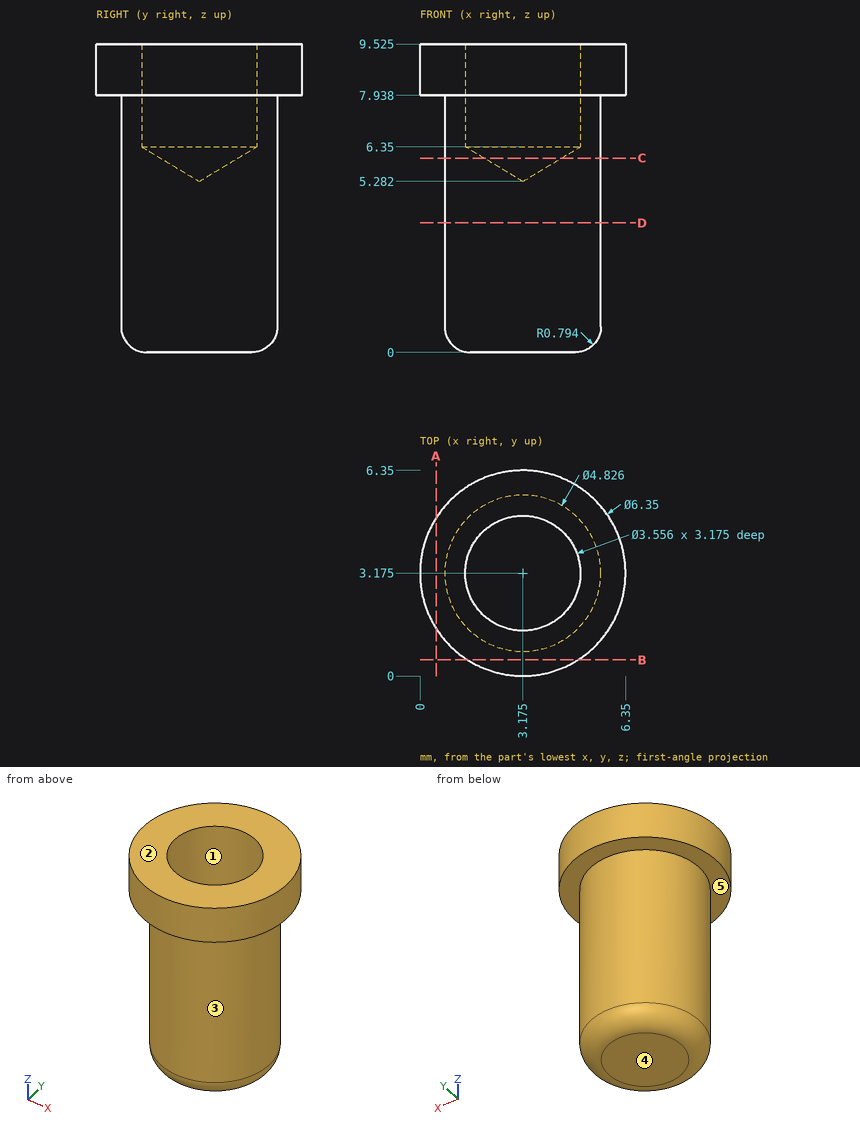
Check sheet for the drawn part. Datum: minimum x, y, z corner. Units: mm. A direction names the side the tool comes from. Round coordinates to 2 decimals unless told otherwise and drop trailing zeros. Loops run counter-clockwise (first coordinate to the right, second up) from the corner with the lowest first, then second, coordinate; pieces in that order, holes last. Notation, with made-up numbers: (-4.75, 58) - (52.25, 58) arc R16 cw to (52.25, 75) - close; hole circle Ø7 at (75.25, 35.25). An arc over 180 degrees is marked (long way). Write item = value, one per line. Start each with the question number.
1. Set-up check for the marked faces 4 and 5: record each of +Z, -Z, +X, -X, +Y, -Y from which the full face is reachable in a straight line by a thin tool's end or side.
2. Section check D-D on z = 4. Enter the section's corners in (x, y) (1 decimal).
3. Mould release check, pull along Y, two halves, no side actions. Record for the marked faces 1, 2 and 3: released by +Y, released by -Y, zero draft, split by the parting line, or undercut.
4. Section check A-A on x = 0.5. Enter the section's corners in (y, z) (1 decimal).
5. Section check C-C on z = 6. Enter the section's corners in (x, y) (1 decimal), then the cut area to 3 significant figures.
6. Thickness scan on line 1 (Z direction, x = 1, y = 5) (1 decimal); line 2 (Y direction, x = 3.25, z = 2.5); line 3 (Y direction, x = 2.5, z = 6.5). Record the ranges inside material, lowest first.
Working result:
q1.face_4 = -Z, +X, -X, +Y, -Y
q1.face_5 = -Z
q2.outline = circle Ø4.8 at (3.2, 3.2)
q3.face_1 = undercut
q3.face_2 = zero draft
q3.face_3 = split by the parting line
q4.outline = (1.5, 7.9) - (4.9, 7.9) - (4.9, 9.5) - (1.5, 9.5) - close
q5.outline = circle Ø4.8 at (3.2, 3.2); hole circle Ø2.4 at (3.2, 3.2)
q5.area = 13.8 mm^2
q6.line_1 = 7.9 to 9.5
q6.line_2 = 0.76 to 5.59
q6.line_3 = 0.86 to 1.53, 4.82 to 5.49
